from build123d import *

# Parameters (mm, degrees)
BOSS_EXTRUDE1_DEPTH = 10
CUT_EXTRUDE4_DEPTH  = 6
SKETCH3_3_R         = 7.5
SKETCH3_3_R_2       = 4.25
SKETCH3_3_R_3       = 1.5
CUT_EXTRUDE5_DEPTH  = 12
SKETCH3_4_R         = 4.25
CUT_EXTRUDE6_DEPTH  = 138.295302177
SKETCH4_R           = 4.25
SKETCH4_W           = 42
SKETCH4_H           = 22
CUT_EXTRUDE8_DEPTH  = 138.295302177
SKETCH5_R           = 11.11
CUT_EXTRUDE10_DEPTH = 8
SKETCH7_W           = 56
SKETCH7_H           = 22.002715538
CUT_EXTRUDE12_DEPTH = 15
SKETCH8_R           = 1.5
CUT_EXTRUDE13_DEPTH = 14
CUT_EXTRUDE14_REACH = 139.295
SKETCH9_R           = 9.5


with BuildPart() as part:
    # Sketch1 → Boss-Extrude1 (new, symmetric)
    with BuildSketch(Plane.XY):
        with BuildLine():
            Line((120, 15), (0, 15))
            ThreePointArc((0, 15), (-15, 0), (0, -15))
            Line((0, -15), (120, -15))
            ThreePointArc((120, -15), (135, 0), (120, 15))
        make_face()
    extrude(amount=BOSS_EXTRUDE1_DEPTH, both=True)

    # Sketch3 → Cut-Extrude4 (cut)
    with BuildSketch(Plane.XY.offset(10)):
        with BuildLine():
            ThreePointArc((90, 4.5), (86.818019485, 3.181980515), (85.5, 0))
            Line((85.5, 0), (94, 0))
            ThreePointArc((94, 0), (94.099918834, 0.538305422), (94.386363636, 1.004895044))
            ThreePointArc((94.386363636, 1.004895044), (92.80427997, 3.519376912), (90, 4.5))
        make_face()
        with BuildLine():
            Line((94, 0), (85.5, 0))
            ThreePointArc((85.5, 0), (86.818019485, -3.181980515), (90, -4.5))
            ThreePointArc((90, -4.5), (92.80427997, -3.519376912), (94.386363636, -1.004895044))
            ThreePointArc((94.386363636, -1.004895044), (94.099918834, -0.538305422), (94, 0))
        make_face()
        with BuildLine():
            Line((118.514851485, 7.351485149), (90, 4.5))
            ThreePointArc((90, 4.5), (92.80427997, 3.519376912), (94.386363636, 1.004895044))
            ThreePointArc((94.386363636, 1.004895044), (96.038305422, 1.400081166), (97, 0))
            ThreePointArc((97, 0), (96.038305422, -1.400081166), (94.386363636, -1.004895044))
            ThreePointArc((94.386363636, -1.004895044), (92.80427997, -3.519376912), (90, -4.5))
            Line((90, -4.5), (118.514851485, -7.351485149))
            ThreePointArc((118.514851485, -7.351485149), (112.5, 0), (118.514851485, 7.351485149))
        make_face()
    extrude(amount=-CUT_EXTRUDE4_DEPTH, mode=Mode.SUBTRACT)

    # Sketch3<3> → Cut-Extrude5 (cut)
    # profile 1 of 2: a face of its own
    with BuildSketch(Plane.XY.offset(10)):
        with Locations((120, 0)):
            Circle(SKETCH3_3_R)
        with Locations((120, 0)):
            Circle(SKETCH3_3_R_2, mode=Mode.SUBTRACT)
    # profile 2 of 2: a face of its own
    with BuildSketch(Plane.XY.offset(10)):
        with Locations((95.5, 0)):
            Circle(SKETCH3_3_R_3)
    extrude(amount=-CUT_EXTRUDE5_DEPTH, mode=Mode.SUBTRACT)

    # Sketch3<4> → Cut-Extrude6 (cut, through all)
    with BuildSketch(Plane.XY.offset(10)):
        with Locations((120, 0)):
            Circle(SKETCH3_4_R)
    extrude(amount=-CUT_EXTRUDE6_DEPTH, mode=Mode.SUBTRACT)

    # Sketch4 → Cut-Extrude8 (cut, through all)
    with BuildSketch(Plane.XY.offset(10)):
        Circle(SKETCH4_R)
        with Locations((38.1, 0)):
            Rectangle(SKETCH4_W, SKETCH4_H)
    extrude(amount=-CUT_EXTRUDE8_DEPTH, mode=Mode.SUBTRACT)

    # Sketch5 → Cut-Extrude10 (cut)
    with BuildSketch(Plane(origin=(0, 0, -10), x_dir=(-1, 0, 0), z_dir=(0, 0, -1))):
        Circle(SKETCH5_R)
    cut_extrude10 = extrude(amount=-CUT_EXTRUDE10_DEPTH, mode=Mode.SUBTRACT)

    # Mirror2: Cut-Extrude10 across plane
    add(cut_extrude10.mirror(Plane.XY), mode=Mode.SUBTRACT)

    # Sketch7 → Cut-Extrude12 (cut)
    with BuildSketch(Plane.XY.offset(10)):
        with Locations((38.1, 0)):
            Rectangle(SKETCH7_W, SKETCH7_H)
    extrude(amount=-CUT_EXTRUDE12_DEPTH, mode=Mode.SUBTRACT)

    # Sketch8 → Cut-Extrude13 (cut)
    with BuildSketch(Plane.XY.offset(-5)):
        with Locations((14.1, 5)):
            Circle(SKETCH8_R)
        with Locations((14.1, -5)):
            Circle(SKETCH8_R)
        with Locations((62.1, -5)):
            Circle(SKETCH8_R)
        with Locations((62.1, 5)):
            Circle(SKETCH8_R)
    extrude(amount=-CUT_EXTRUDE13_DEPTH, mode=Mode.SUBTRACT)

    # Cut-Extrude14: up to this face of the body (flat: up to its plane)
    cut_extrude14_end = Plane(part.part.faces().sort_by_distance((112.712132034, 0, -2))[0])
    # Sketch9 → Cut-Extrude14 (cut, up to the picked face)
    with BuildSketch(Plane.XY.offset(10), mode=Mode.PRIVATE) as cut_extrude14_sk1:
        with Locations((120, 0)):
            Circle(SKETCH9_R)
    cut_extrude14_tool1 = split(extrude(cut_extrude14_sk1.sketch, amount=-CUT_EXTRUDE14_REACH, mode=Mode.PRIVATE), bisect_by=cut_extrude14_end, keep=Keep.BOTH, mode=Mode.PRIVATE)
    add(cut_extrude14_tool1.solids().sort_by(Axis((120, 0, 10), (0, 0, -1)))[0], mode=Mode.SUBTRACT)


solid = part.part
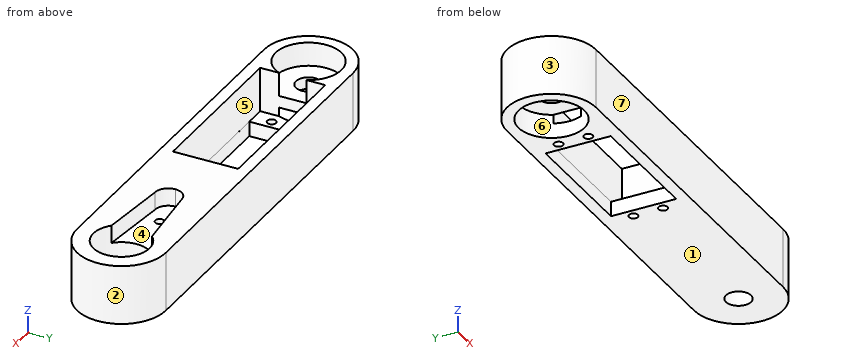
Could you check a few things on this model? Use its own coordinates, in mm. Face numbers are marked on the shaded views. A direction names the side the tool comes from. Coordinates: 2 decimals unless noted, no trailing zeros. Write each loop counter-clockwise with the first axis right and the second up, starting at its lowest first coordinate (ties: lowest second). Pieces come first, ordered by that corner, then holes. Notation, with made-up numbers: (-29.5, 13) - (26.5, 13) arc R9 cw to (26.5, 23) - close; hole circle Ø7 at (11, 61). An arc over 180 degrees is marked (long way). Put each result on its own line as item: value. Start each with the question number.
Q1. I want a section at A-A on x = 62.1. Write out the boundary of the cut face in (y, z), plus the area to 3 significant figures.
Q2. I'm going to push flat-ended pins straight in: P1, Ø5, axis at x = 62.1, y = -5, coming from the +Z side; P2, Ø4.5, axis at y = -4.5, z = -0.5, coming from the -X side; P3, Ø7.5, axis at y = 1, z = 2, coming from the +X side; P4, Ø18, axis at x = 0, y = 0, coming from the +Z side. Where does each tip first touch, or does it pass through?
Q3. Thinking about a two-plate mould opening in X: for the marked faces 1, 2, 3 and 4, which applies, pulls with the +X half, pulls with the -X half, needs draft (parallel to the pull), parting line crosses it, or undercut?
Q4. Please list where these lines run through material, in increasing order: L1, parallel to Y at x = 62.1, z = -6.6; L2, parallel to X at y = 0.5, z = 4.25; L3, parallel to X at y = -2, z = 7.25.
Q5. I want a section at B-B on z = -0.5. Write out the boundary of the cut face in (x, y), plus the area to 3 significant figures.
Q6. Which directions (+Z, -Z, +X, -X, +Y, -Y) give clear straight access to the entire face, cutting with the end or side of a thin tool? Please do the marked faces 5, 6 and 7.
Q7. I want a section at C-C on z = 7. Write out the boundary of the cut face in (x, y), plus the area to 3 significant figures.
Checks:
1. outline: (-15, -10) - (-6.5, -10) - (-6.5, -5) - (-11, -5) - (-11, 10) - (-15, 10) - close; (-3.5, -10) - (3.5, -10) - (3.5, -5) - (-3.5, -5) - close; (6.5, -10) - (15, -10) - (15, 10) - (11, 10) - (11, -5) - (6.5, -5) - close
1. area: 240 mm²
2. P1: z = -5
2. P2: x = -14.83
2. P3: x = 135
2. P4: z = 2
3. face 1: needs draft
3. face 2: pulls with the +X half
3. face 3: pulls with the -X half
3. face 4: undercut
4. L1: -15 to -6.5, -3.5 to 3.5, 6.5 to 15
4. L2: -14.99 to -11.1, 66.1 to 85.53, 129.49 to 134.99
4. L3: -14.87 to -10.93, 66.1 to 85.97, 129.29 to 134.87
5. outline: (0, -15) - (120, -15) arc R15 ccw to (120, 15) - (0, 15) arc R15 ccw to start; hole circle Ø8.5 at (0, 0); hole (10.1, -11) - (66.1, -11) - (66.1, 11) - (10.1, 11) - close; hole circle Ø3 at (95.5, 0); hole circle Ø19 at (120, 0)
5. area: 2,730 mm²
6. face 5: +Z
6. face 6: -Z
6. face 7: +Z, -Z, +X, -X, -Y
7. outline: (0, -15) - (120, -15) arc R15 ccw to (120, 15) - (0, 15) arc R15 ccw to start; hole (10.1, -11) - (66.1, -11) - (66.1, 11) - (10.1, 11) - (10.1, 4.63) arc R11.11 ccw (long way) to (10.1, -4.63) - close; hole (90, -4.5) - (113.41, -6.84) arc R9.5 ccw (long way) to (113.41, 6.84) - (90, 4.5) arc R4.5 ccw to start
7. area: 2,140 mm²
